Geometry check sheet. Reference: drawing and pictorial views, mm from the part's lowest x, y, z. Round coordinates to 2 decimals unless told otherwise and drop trailing zeros. Loops run counter-clockwise (first coordinate to the right, second up) from the corner with the lowest first, then second, coordinate; pieces in that order, holes last. Notation, with made-up numbers: (11, -36.75) - (40, -36.75) arc R28 cw to (40, -10.75) - close; hole circle Ø1 at (74.5, -26.75). An arc over 180 degrees is marked (long way). Return JSON: item names as keys, results as strings.
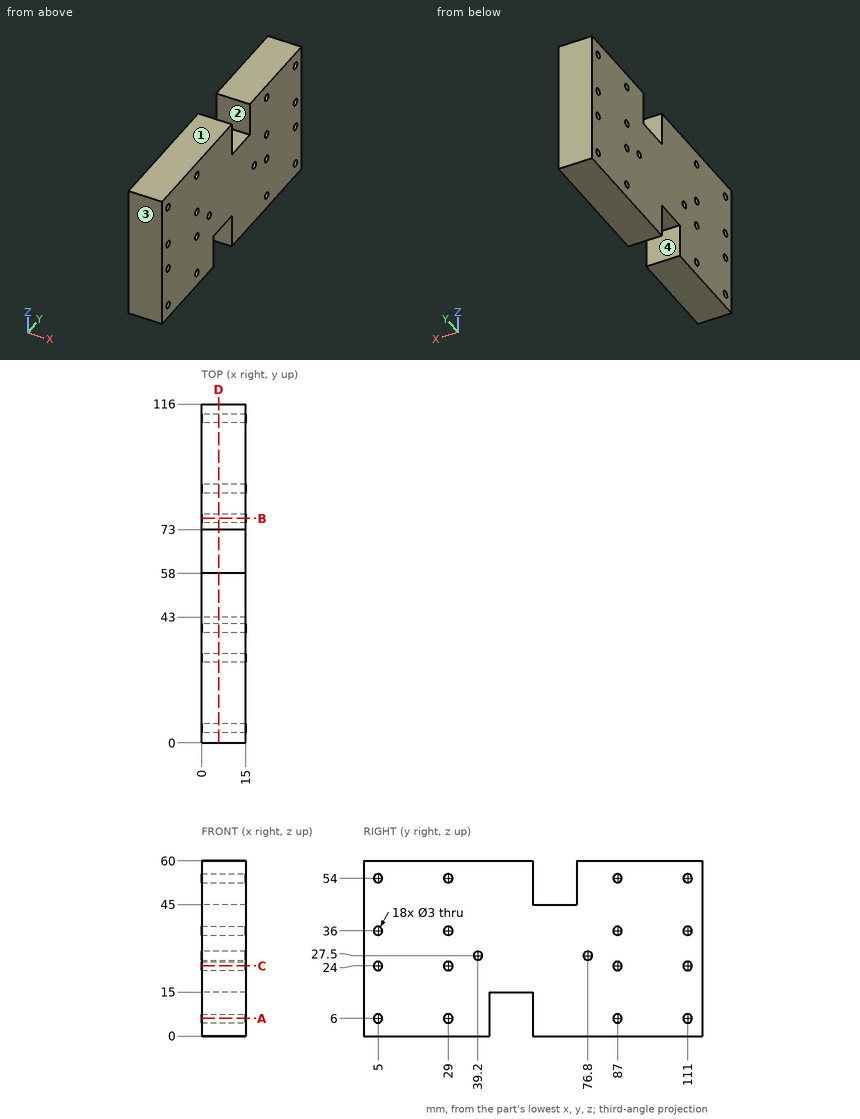
Q1. Depth check by flat-ended pin: P1, Ø2.5, axis at y = 29, z = 54, coming from the +X side; P2, Ø7.5, axis at x = 10, y = 53.5, coming from the -Z side. Enter the tip coordinate at first touch or a pass-through.
Answer key:
{"P1": "passes through", "P2": "stops at z = 15"}
Q2. Draft check along Y on the marked faces 1, 2, 3 and 4. Enter one of: released by +Y, released by -Y, zero draft, split by the parting line, or undercut.
Answer key:
{"face 1": "zero draft", "face 2": "undercut", "face 3": "released by -Y", "face 4": "undercut"}
Q3. Sectioned sample at B-B (y = 76.8). Enter the section's corners in (x, z).
Answer key:
{"outline": "(0, 0) - (15, 0) - (15, 26) - (0, 26) - close; (0, 29) - (15, 29) - (15, 60) - (0, 60) - close"}
Q4. Scan lines: probe 1 along Y at (x, z) = (4, 24); probe 2 along Y at (x, z) = (7, 54); probe 3 along Y at (x, z) = (12, 6). Record each from-to range of solid material in increasing order. Write a range as [from, to].
Answer key:
{"probe 1": "y = [0, 3.5], [6.5, 27.5], [30.5, 85.5], [88.5, 109.5], [112.5, 116]", "probe 2": "y = [0, 3.5], [6.5, 27.5], [30.5, 58], [73, 85.5], [88.5, 109.5], [112.5, 116]", "probe 3": "y = [0, 3.5], [6.5, 27.5], [30.5, 43], [58, 85.5], [88.5, 109.5], [112.5, 116]"}
Q5. Sectioned sample at C-C (z = 24). Enter the section's corners in (x, y).
Answer key:
{"outline": "(0, 0) - (15, 0) - (15, 3.5) - (0, 3.5) - close; (0, 6.5) - (15, 6.5) - (15, 27.5) - (0, 27.5) - close; (0, 30.5) - (15, 30.5) - (15, 85.5) - (0, 85.5) - close; (0, 88.5) - (15, 88.5) - (15, 109.5) - (0, 109.5) - close; (0, 112.5) - (15, 112.5) - (15, 116) - (0, 116) - close"}
Q6. Sectioned sample at D-D (x = 5.75). State how many separate pieces and enclosed holes the cut face has, plus the area to 3 significant figures.
Answer key:
{"separate pieces": "1", "enclosed holes": "18", "area": "6,380 mm²"}
Q7. Sectioned sample at A-A (z = 6). Enter the section's corners in (x, y), plus the area to 4 significant figures.
Answer key:
{"outline": "(0, 0) - (15, 0) - (15, 3.5) - (0, 3.5) - close; (0, 6.5) - (15, 6.5) - (15, 27.5) - (0, 27.5) - close; (0, 30.5) - (15, 30.5) - (15, 43) - (0, 43) - close; (0, 58) - (15, 58) - (15, 85.5) - (0, 85.5) - close; (0, 88.5) - (15, 88.5) - (15, 109.5) - (0, 109.5) - close; (0, 112.5) - (15, 112.5) - (15, 116) - (0, 116) - close", "area": "1,335 mm²"}
